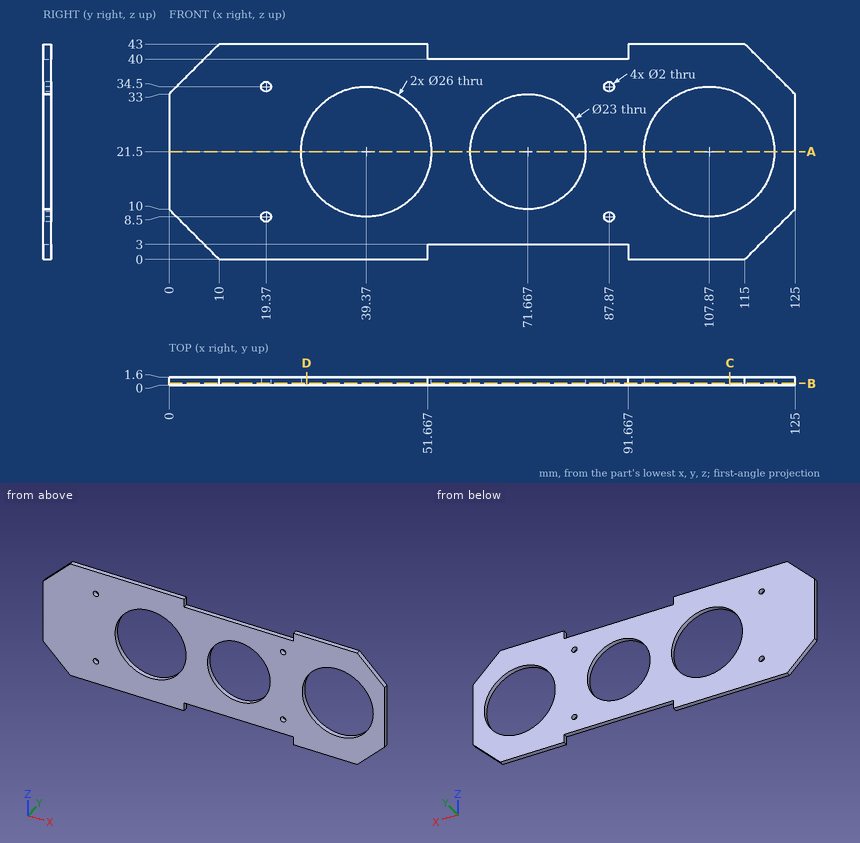
For this review, use the dimensioned drawing (mm, ordinates from the lowest corner) and the shaded views. Round coordinates to 2 decimals unless told otherwise and drop trailing zeros. Order: outer loops, then holes, each group sorted by start corner. A loop starts at its lowest first (then second) coordinate and runs counter-clockwise, first axis right, second up. Notation, with made-up numbers: (-32, 53) -> (-23, 53) arc R20 ccw to (-23, 57) -> close; hole circle Ø2 at (11.5, 19). An arc over 180 degrees is marked (long way). Write item = value, one per line. Start each with the question number.
Item 1: Consider section D-D on x = 27.5. Write out the cut boundary in (y, z).
Item 2: Consider section B-B on y = 0.4. Write out the cut boundary in (x, z).
Item 3: Consider section C-C on x = 112. Write out the cut boundary in (y, z).
Item 4: Consider section A-A on z = 21.5. Write out the cut boundary in (x, y).
Item 5: For line 1 along X through (y, z) = (0.75, 21.5); line 2 along Z through (x, y) = (19.5, 0.9); line 3 along X through (y, z) = (0.35, 31.5) (1 decimal), list the stretches that pass through material, from the lowest coordinate up.
Item 6: Clearance check with flat-ended pins moving along their axes: pin 1 Ø18.5 at (x, z) = (71.67, 21.5) entering from +Y; pin 2 Ø0.5 at (y, z) = (0.5, 1) entering from +X; pin 3 Ø0.5 at (x, y) = (77, 0.5) entering from +Z; pin 4 Ø0.5 at (y, z) = (0.5, 2) entering from -X. State where each tip first meets the part, or that it passes through.
Conclusion:
q1.outline = (0, 0) -> (1.6, 0) -> (1.6, 16.2) -> (0, 16.2) -> close; (0, 26.8) -> (1.6, 26.8) -> (1.6, 43) -> (0, 43) -> close
q2.outline = (0, 10) -> (10, 0) -> (51.67, 0) -> (51.67, 3) -> (91.67, 3) -> (91.67, 0) -> (115, 0) -> (125, 10) -> (125, 33) -> (115, 43) -> (91.67, 43) -> (91.67, 40) -> (51.67, 40) -> (51.67, 43) -> (10, 43) -> (0, 33) -> close; hole circle Ø2 at (19.37, 8.5); hole circle Ø2 at (19.37, 34.5); hole circle Ø26 at (39.37, 21.5); hole circle Ø23 at (71.67, 21.5); hole circle Ø2 at (87.87, 8.5); hole circle Ø2 at (87.87, 34.5); hole circle Ø26 at (107.87, 21.5)
q3.outline = (0, 0) -> (1.6, 0) -> (1.6, 9.17) -> (0, 9.17) -> close; (0, 33.83) -> (1.6, 33.83) -> (1.6, 43) -> (0, 43) -> close
q4.outline = (0, 0) -> (26.37, 0) -> (26.37, 1.6) -> (0, 1.6) -> close; (52.37, 0) -> (60.17, 0) -> (60.17, 1.6) -> (52.37, 1.6) -> close; (83.17, 0) -> (94.87, 0) -> (94.87, 1.6) -> (83.17, 1.6) -> close; (120.87, 0) -> (125, 0) -> (125, 1.6) -> (120.87, 1.6) -> close
q5.line_1 = 0 to 26.37, 52.37 to 60.17, 83.17 to 94.87, 120.87 to 125
q5.line_2 = 0 to 7.51, 9.49 to 33.51, 35.49 to 43
q5.line_3 = 0 to 31.1, 47.7 to 66, 77.3 to 99.6, 116.2 to 125
q6.pin_1 = through
q6.pin_2 = 116.25
q6.pin_3 = 40
q6.pin_4 = 7.75
